Input: part model. Units: mm. Frame: model coordinates. A direction names the side the tool comes from. Give positions to 0.01 mm unless a question says otherwise; leave off trailing zeros. Write each loop counter-clockwise with the first axis right and the second up, starting at its lowest first coordinate (ties: lowest second). Pieces come first, ordered by that corner, then holes. Notation, with made-up numbers: (38.5, 55.5) - (59.5, 55.5) arc R13 ccw to (59.5, 67.5) - close; hole circle Ø10 at (0.25, 27.5). An arc over 180 degrees is marked (long way). Use a Markdown table: item, result. Add a question column.
1. Material intervals for probe 1 along Y at (x, z) = (27, 10); probe 2 along X at (y, z) = (-107.5, 7.5) (3 decimals); probe 3 along X at (y, z) = (-119.05, 7.5) (3 decimals), sorted ascending.
2. Set-up query: faces 1 (the flat face through (11.9, -0.2, 9.5)), 2 (the flat face through (-7, -30.4, 11)), 3 (the flat face through (-4, -100.4, 8)). Return all of +Z, -Z, +X, -X, +Y, -Y with unobstructed straight access to the full face (end or side cutting, diameter ignored); none if empty.
3. Section query A-A, the plane y = -8.4. Return loops of the section in (x, z) (3 decimals).
4. Mould query, pull axis Z, two halves, no side actions, for faces 4 (the flat face through (11, -69, 0)), 5 (the cylindrical face through (-3.81, -106.46, 8.95)), 6 (the cylindrical face through (20.98, -8.99, 11.2)), 7 (the cylindrical face through (26.01, -106.46, 7.81)). Classes: released by +Z, released by -Z, zero draft, split by the parting line, or undercut.
5. Pin query (flat end, axial travel): pin 1 (4.5 mm diameter, centred on x = 27.425, z = 7.5, fed in from -Y); pin 2 (6 mm diameter, centred on y = -88, z = 6.5, fed in from +X); pin 3 (1.5 mm diameter, centred on x = 30, z = 3.5, fed in from +Y); pin 4 (3.5 mm diameter, centred on x = -6.835, z = 3.75, fed in from +Y). Return the tip coordinate at first contact, or that it passes through.
6. Section query B-B, the plane y = -54. Return loops of the section in (x, z), plus the area to 3 significant figures.
7. Section query C-C, the plane y = -89. Return loops of the section in (x, z).
```python
from build123d import *

# Parameters (mm, degrees)
SKETCH_1_R          = 1.55
EXTRUDE_1_DEPTH     = 15
CUT_EXTRUDE_1_DEPTH = 18.2
SKETCH_3_R          = 1.5
CUT_EXTRUDE_2_DEPTH = 12
SKETCH_4_R          = 1.5
CUT_EXTRUDE_3_DEPTH = 12
CHAMFER_1_SIZE      = 1
CUT_EXTRUDE_4_DEPTH = 9.5
CUT_EXTRUDE_5_DEPTH = 9.5
SKETCH_7_R          = 1.45
CUT_EXTRUDE_6_DEPTH = 20


with BuildPart() as part:
    # 草图1 → 凸台-拉伸1 (new body)
    with BuildSketch(Plane.XY):
        with BuildLine():
            Line((-10.835, -18.4), (-9.52124, -120.4))
            Line((-9.52124, -120.4), (1.775, -120.4))
            ThreePointArc((1.775, -120.4), (11.775, -110.4), (21.775, -120.4))
            Line((21.775, -120.4), (33.07124, -120.4))
            Line((33.07124, -120.4), (34.385, -18.4))
            Line((34.385, -18.4), (26.795, -18.4))
            Line((26.795, -18.4), (26.595, -18.4))
            Line((26.595, -18.4), (23.385271739, -0.2))
            Line((23.385271739, -0.2), (0.164728261, -0.2))
            Line((0.164728261, -0.2), (-3.045, -18.4))
            Line((-3.045, -18.4), (-3.245, -18.4))
            Line((-3.245, -18.4), (-10.835, -18.4))
        make_face()
        with Locations((4.005, -8.4)):
            Circle(SKETCH_1_R, mode=Mode.SUBTRACT)
        with Locations((19.545, -8.4)):
            Circle(SKETCH_1_R, mode=Mode.SUBTRACT)
    extrude(amount=EXTRUDE_1_DEPTH)

    # 草图2 → 切除-拉伸1 (cut)
    with BuildSketch(Plane(origin=(0, -0.2, 0), x_dir=(1, 0, 0), z_dir=(0, 1, 0))):
        Polygon((23.385271739, -7.5), (-22.23859784, -7.5), (-22.23859784, 0), (39.198950906, 0), (39.198950906, -7.5), align=None)
    extrude(amount=-CUT_EXTRUDE_1_DEPTH, mode=Mode.SUBTRACT)

    # 草图3 → 切除-拉伸2 (cut)
    with BuildSketch(Plane(origin=(0, -0.2, 0), x_dir=(1, 0, 0), z_dir=(0, 1, 0))):
        with Locations(Location((11.775, -11.25, 0), (0, 0, 270))):
            Circle(SKETCH_3_R)
    extrude(amount=-CUT_EXTRUDE_2_DEPTH, mode=Mode.SUBTRACT)

    # 草图4 → 切除-拉伸3 (cut)
    with BuildSketch(Plane(origin=(0, -18.4, 0), x_dir=(1, 0, 0), z_dir=(0, 1, 0))):
        with Locations(Location((30.385, -3.75, 0), (0, 0, 180))):
            Circle(SKETCH_4_R)
        with Locations(Location((30.385, -11.25, 0), (0, 0, 180))):
            Circle(SKETCH_4_R)
        with Locations((-6.835, -11.25)):
            Circle(SKETCH_4_R)
        with Locations((-6.835, -3.75)):
            Circle(SKETCH_4_R)
    extrude(amount=-CUT_EXTRUDE_3_DEPTH, mode=Mode.SUBTRACT)

    # 倒角1
    chamfer_1_edges = [part.edges().sort_by_distance(p)[0] for p in [
        (33.72812, -69.4, 15),
        (-10.17812, -69.4, 0),
        (33.72812, -69.4, 0),
        (-10.17812, -69.4, 15),
    ]]
    chamfer(chamfer_1_edges, length=CHAMFER_1_SIZE)

    # 草图5 → 切除-拉伸4 (cut)
    with BuildSketch(Plane(origin=(34.616249358, -0.445857292, 0), x_dir=(0, 0, -1), z_dir=(0.9999170631189305, -0.012878931772971664, 0))):
        Polygon((-7.5, -114.964092156), (-4.75, -114.964092156), (-4.75, -111.964092156), (-10.25, -111.964092156), (-10.25, -114.964092156), align=None)
    extrude(amount=-CUT_EXTRUDE_4_DEPTH, mode=Mode.SUBTRACT)

    # 草图6 → 切除-拉伸5 (cut)
    with BuildSketch(Plane(origin=(-11.070155523, -0.142583603, 0), x_dir=(0, 0, 1), z_dir=(-0.9999170631189305, -0.012878931772971934, 0))):
        Polygon((7.5, -115.267390999), (4.75, -115.267390999), (4.75, -112.267390999), (10.25, -112.267390999), (10.25, -115.267390999), align=None)
    extrude(amount=-CUT_EXTRUDE_5_DEPTH, mode=Mode.SUBTRACT)

    # 草图7 → 切除-拉伸6 (cut)
    with BuildSketch(Plane.XZ.offset(120.4)):
        with Locations(Location((27.425, 7.5, 0), (0, 0, 270))):
            Circle(SKETCH_7_R)
        with Locations(Location((-3.875, 7.5, 0), (0, 0, 270))):
            Circle(SKETCH_7_R)
    extrude(amount=-CUT_EXTRUDE_6_DEPTH, mode=Mode.SUBTRACT)


solid = part.part
```
Result sheet:
| question | item | result |
|---|---|---|
| 1 | probe 1 | y = -120.4 to -115.32, -112.32 to -18.4 |
| 1 | probe 2 | x = -9.687 to -5.325, -2.425 to 25.975, 28.875 to 33.237 |
| 1 | probe 3 | x = -9.539 to -5.325, -2.425 to 1.867, 21.683 to 25.975, 28.875 to 33.089 |
| 2 | face 1 | +Z, -Z, +X, -X, +Y |
| 2 | face 2 | +Y |
| 2 | face 3 | -Y |
| 3 | outline | (-1.281, 7.5) - (2.455, 7.5) - (2.455, 15) - (-1.281, 15) - close; (5.555, 7.5) - (17.995, 7.5) - (17.995, 15) - (5.555, 15) - close; (21.095, 7.5) - (24.831, 7.5) - (24.831, 15) - (21.095, 15) - close; hole circle Ø3 at (11.775, 11.25) |
| 4 | face 4 | released by -Z |
| 4 | face 5 | undercut |
| 4 | face 6 | zero draft |
| 4 | face 7 | undercut |
| 5 | pin 1 | stops at y = -120.4 |
| 5 | pin 2 | stops at x = 33.53 |
| 5 | pin 3 | stops at y = -30.4 |
| 5 | pin 4 | stops at y = -18.4 |
| 6 | outline | (-10.38, 1) - (-9.38, 0) - (32.93, 0) - (33.93, 1) - (33.93, 14) - (32.93, 15) - (-9.38, 15) - (-10.38, 14) - close |
| 6 | area | 663 mm² |
| 7 | outline | (-9.93, 1) - (-8.93, 0) - (32.48, 0) - (33.48, 1) - (33.48, 14) - (32.48, 15) - (-8.93, 15) - (-9.93, 14) - close |
